from build123d import *

# Parameters (mm, degrees)
SKICA1_W                  = 100
SKICA1_H                  = 100
P_IDAT_VYSUNUT_M1_DEPTH   = 3
SKICA2_R                  = 1.5
ODEBRAT_VYSUNUT_M5_DEPTH  = 3
SKICA3_W                  = 75
SKICA3_H                  = 2
P_IDAT_VYSUNUT_M4_DEPTH   = 53
SKICA10_W                 = 8
SKICA10_H                 = 2
ODEBRAT_VYSUNUT_M6_DEPTH  = 50
SKICA11_W                 = 10
SKICA11_H                 = 2
ODEBRAT_VYSUNUT_M8_DEPTH  = 15
SKICA16_W                 = 67
SKICA16_H                 = 2
P_IDAT_VYSUNUT_M6_DEPTH   = 15
SKICA17_W                 = 2.5
SKICA17_H                 = 2.5
P_IDAT_VYSUNUT_M7_DEPTH   = 15
SKICA18_W                 = 2.5
SKICA18_H                 = 2.5
P_IDAT_VYSUNUT_M8_DEPTH   = 15
SKICA19_W                 = 1
SKICA19_H                 = 1
P_IDAT_VYSUNUT_M10_DEPTH  = 50
SKICA20_W                 = 1
SKICA20_H                 = 1
P_IDAT_VYSUNUT_M11_DEPTH  = 35
SKICA21_W                 = 1
SKICA21_H                 = 1
P_IDAT_VYSUNUT_M12_DEPTH  = 35
SKICA22_W                 = 1
SKICA22_H                 = 1
P_IDAT_VYSUNUT_M13_DEPTH  = 50
SKICA24_W                 = 91
SKICA24_H                 = 2
P_IDAT_VYSUNUT_M14_DEPTH  = 15
SKICA25_W                 = 2
SKICA25_H                 = 2
P_IDAT_VYSUNUT_M15_DEPTH  = 35
SKICA26_W                 = 2
SKICA26_H                 = 2
P_IDAT_VYSUNUT_M16_DEPTH  = 35
SKICA27_W                 = 2
SKICA27_H                 = 49.75
P_IDAT_VYSUNUT_M17_DEPTH  = 15
SKICA28_W                 = 100
SKICA28_H                 = 5
P_IDAT_VYSUNUT_M18_DEPTH  = 5
SKICA30_W                 = 5
SKICA30_H                 = 90
P_IDAT_VYSUNUT_M19_DEPTH  = 5
SKICA31_W                 = 100
SKICA31_H                 = 100
ODEBRAT_VYSUNUT_M9_DEPTH  = 6
SKICA32_W                 = 2
SKICA32_H                 = 15
ODEBRAT_VYSUNUT_M10_DEPTH = 6
SKICA33_W                 = 2
SKICA33_H                 = 23
P_IDAT_VYSUNUT_M22_DEPTH  = 25
P_IDAT_VYSUNUT_M23_DEPTH  = 10
SKICA35_W                 = 50
SKICA35_H                 = 2
P_IDAT_VYSUNUT_M24_DEPTH  = 10
SKICA36_W                 = 2
SKICA36_H                 = 45
P_IDAT_VYSUNUT_M25_DEPTH  = 2
SKICA37_W                 = 2
SKICA37_H                 = 2
P_IDAT_VYSUNUT_M26_DEPTH  = 60
SKICA38_W                 = 10
SKICA38_H                 = 1
P_IDAT_VYSUNUT_M27_DEPTH  = 35
SKICA40_W                 = 2
SKICA40_H                 = 2
P_IDAT_VYSUNUT_M29_DEPTH  = 35


with BuildPart() as part:
    # Skica1 → Přidat vysunutím1 (new body)
    with BuildSketch(Plane(origin=(0, 0, 0), x_dir=(1, 0, 0), z_dir=(0, 1, 0))):
        Rectangle(SKICA1_W, SKICA1_H)
    extrude(amount=P_IDAT_VYSUNUT_M1_DEPTH)

    # Skica2 → Odebrat vysunutím5 (cut)
    with BuildSketch(Plane(origin=(0, 0, 0), x_dir=(1, 0, 0), z_dir=(0, 1, 0))):
        with Locations((-18, 40)):
            Circle(SKICA2_R)
        with Locations((40, 40)):
            Circle(SKICA2_R)
        with Locations((40, -8.5)):
            Circle(SKICA2_R)
        with Locations((-18, -8.5)):
            Circle(SKICA2_R)
    extrude(amount=ODEBRAT_VYSUNUT_M5_DEPTH, mode=Mode.SUBTRACT)

    # Skica3 → Přidat vysunutím4 (add)
    with BuildSketch(Plane(origin=(0, 0, 0), x_dir=(1, 0, 0), z_dir=(0, 1, 0))):
        Polygon((40, 50), (40, 48), (48, 48), (48, 27.25), (50, 27.25), (50, 50), align=None)
        Polygon((-50, -20), (-48, -20), (-48, -48), (48, -48), (48, 4.25), (50, 4.25), (50, -50), (-50, -50), align=None)
        with Locations((-12.5, 49)):
            Rectangle(SKICA3_W, SKICA3_H)
    extrude(amount=P_IDAT_VYSUNUT_M4_DEPTH)

    # Skica10 → Odebrat vysunutím6 (cut)
    with BuildSketch(Plane(origin=(0, 53, 0), x_dir=(1, 0, 0), z_dir=(0, 1, 0))):
        with Locations((21, 49)):
            Rectangle(SKICA10_W, SKICA10_H)
    extrude(amount=-ODEBRAT_VYSUNUT_M6_DEPTH, mode=Mode.SUBTRACT)

    # Skica11 → Odebrat vysunutím8 (cut)
    with BuildSketch(Plane(origin=(0, 53, 0), x_dir=(1, 0, 0), z_dir=(0, 1, 0))):
        with Locations((-32, -49)):
            Rectangle(SKICA11_W, SKICA11_H)
        with Locations((-11, -49)):
            Rectangle(SKICA11_W, SKICA11_H)
        with Locations((10, -49)):
            Rectangle(SKICA11_W, SKICA11_H)
        with Locations((31, -49)):
            Rectangle(SKICA11_W, SKICA11_H)
    extrude(amount=-ODEBRAT_VYSUNUT_M8_DEPTH, mode=Mode.SUBTRACT)

    # Skica16 → Přidat vysunutím6 (add)
    with BuildSketch(Plane(origin=(0, 3, 0), x_dir=(1, 0, 0), z_dir=(0, 1, 0))):
        with Locations((-16.5, 47)):
            Rectangle(SKICA16_W, SKICA16_H)
    extrude(amount=P_IDAT_VYSUNUT_M6_DEPTH)

    # Skica17 → Přidat vysunutím7 (add)
    with BuildSketch(Plane(origin=(0, 3, 0), x_dir=(1, 0, 0), z_dir=(0, 1, 0))):
        with Locations((46.75, -46.75)):
            Rectangle(SKICA17_W, SKICA17_H)
    extrude(amount=P_IDAT_VYSUNUT_M7_DEPTH)

    # Skica18 → Přidat vysunutím8 (add)
    with BuildSketch(Plane(origin=(0, 3, 0), x_dir=(1, 0, 0), z_dir=(0, 1, 0))):
        with Locations((-46.75, -46.75)):
            Rectangle(SKICA18_W, SKICA18_H)
    extrude(amount=P_IDAT_VYSUNUT_M8_DEPTH)

    # Skica19 → Přidat vysunutím10 (add)
    with BuildSketch(Plane(origin=(0, 3, 0), x_dir=(1, 0, 0), z_dir=(0, 1, 0))):
        with Locations((47.5, 47.5)):
            Rectangle(SKICA19_W, SKICA19_H)
    extrude(amount=P_IDAT_VYSUNUT_M10_DEPTH)

    # Skica20 → Přidat vysunutím11 (add)
    with BuildSketch(Plane(origin=(0, 18, 0), x_dir=(1, 0, 0), z_dir=(0, 1, 0))):
        with Locations((47.5, -47.5)):
            Rectangle(SKICA20_W, SKICA20_H)
    extrude(amount=P_IDAT_VYSUNUT_M11_DEPTH)

    # Skica21 → Přidat vysunutím12 (add)
    with BuildSketch(Plane(origin=(0, 18, 0), x_dir=(1, 0, 0), z_dir=(0, 1, 0))):
        with Locations((-47.5, -47.5)):
            Rectangle(SKICA21_W, SKICA21_H)
    extrude(amount=P_IDAT_VYSUNUT_M12_DEPTH)

    # Skica22 → Přidat vysunutím13 (add)
    with BuildSketch(Plane(origin=(0, 3, 0), x_dir=(1, 0, 0), z_dir=(0, 1, 0))):
        with Locations((-47.5, -20.5)):
            Rectangle(SKICA22_W, SKICA22_H)
    extrude(amount=P_IDAT_VYSUNUT_M13_DEPTH)

    # Skica24 → Přidat vysunutím14 (add)
    with BuildSketch(Plane(origin=(0, 3, 0), x_dir=(1, 0, 0), z_dir=(0, 1, 0))):
        with Locations((0, -47)):
            Rectangle(SKICA24_W, SKICA24_H)
    extrude(amount=P_IDAT_VYSUNUT_M14_DEPTH)

    # Skica25 → Přidat vysunutím15 (add)
    with BuildSketch(Plane(origin=(0, 18, 0), x_dir=(1, 0, 0), z_dir=(0, 1, 0))):
        with Locations((20.5, -47)):
            Rectangle(SKICA25_W, SKICA25_H)
        with Locations((-0.5, -47)):
            Rectangle(SKICA25_W, SKICA25_H)
        with Locations((-21.5, -47)):
            Rectangle(SKICA25_W, SKICA25_H)
    extrude(amount=P_IDAT_VYSUNUT_M15_DEPTH)

    # Skica26 → Přidat vysunutím16 (add)
    with BuildSketch(Plane(origin=(0, 18, 0), x_dir=(1, 0, 0), z_dir=(0, 1, 0))):
        with Locations((-49, 47)):
            Rectangle(SKICA26_W, SKICA26_H)
        with Locations((16, 47)):
            Rectangle(SKICA26_W, SKICA26_H)
    extrude(amount=P_IDAT_VYSUNUT_M16_DEPTH)

    # Skica27 → Přidat vysunutím17 (add)
    with BuildSketch(Plane(origin=(0, 3, 0), x_dir=(1, 0, 0), z_dir=(0, 1, 0))):
        with Locations((47, -20.625)):
            Rectangle(SKICA27_W, SKICA27_H)
    extrude(amount=P_IDAT_VYSUNUT_M17_DEPTH)

    # Skica28 → Přidat vysunutím18 (add)
    with BuildSketch(Plane(origin=(0, 0, 0), x_dir=(1, 0, 0), z_dir=(0, 1, 0))):
        with Locations((0, -47.5)):
            Rectangle(SKICA28_W, SKICA28_H)
        with Locations((0, 47.5)):
            Rectangle(SKICA28_W, SKICA28_H)
    extrude(amount=-P_IDAT_VYSUNUT_M18_DEPTH)

    # Skica30 → Přidat vysunutím19 (add)
    with BuildSketch(Plane(origin=(0, 0, 0), x_dir=(-1, 0, 0), z_dir=(0, -1, 0))):
        with Locations((47.5, 0)):
            Rectangle(SKICA30_W, SKICA30_H)
        with Locations((-47.5, 0)):
            Rectangle(SKICA30_W, SKICA30_H)
    extrude(amount=P_IDAT_VYSUNUT_M19_DEPTH)

    # Skica31 → Odebrat vysunutím9 (cut)
    with BuildSketch(Plane(origin=(0, -5, 0), x_dir=(-1, 0, 0), z_dir=(0, -1, 0))):
        Rectangle(SKICA31_W, SKICA31_H)
    extrude(amount=-ODEBRAT_VYSUNUT_M9_DEPTH, mode=Mode.SUBTRACT)

    # Skica32 → Odebrat vysunutím10 (cut)
    with BuildSketch(Plane.ZY.offset(-15)):
        with Locations((-47, 45.5)):
            Rectangle(SKICA32_W, SKICA32_H)
    extrude(amount=-ODEBRAT_VYSUNUT_M10_DEPTH, mode=Mode.SUBTRACT)

    # Skica33 → Přidat vysunutím22 (add)
    with BuildSketch(Plane(origin=(0, 3, 0), x_dir=(1, 0, 0), z_dir=(0, 1, 0))):
        with Locations((49, 15.75)):
            Rectangle(SKICA33_W, SKICA33_H)
    extrude(amount=P_IDAT_VYSUNUT_M22_DEPTH)

    # Skica34 → Přidat vysunutím23 (add)
    with BuildSketch(Plane(origin=(0, 53, 0), x_dir=(1, 0, 0), z_dir=(0, 1, 0))):
        Polygon((40, 50), (50, 50), (50, 27.25), (48, 27.25), (48, 47), (47, 47), (47, 48), (40, 48), align=None)
    extrude(amount=P_IDAT_VYSUNUT_M23_DEPTH)

    # Skica35 → Přidat vysunutím24 (add)
    with BuildSketch(Plane(origin=(0, 53, 0), x_dir=(1, 0, 0), z_dir=(0, 1, 0))):
        with Locations((-8, 49)):
            Rectangle(SKICA35_W, SKICA35_H)
    extrude(amount=P_IDAT_VYSUNUT_M24_DEPTH)

    # Skica36 → Přidat vysunutím25 (add)
    with BuildSketch(Plane.XY.offset(-48)):
        with Locations((-32, 40.5)):
            Rectangle(SKICA36_W, SKICA36_H)
    extrude(amount=P_IDAT_VYSUNUT_M25_DEPTH)

    # Skica37 → Přidat vysunutím26 (add)
    with BuildSketch(Plane(origin=(0, 3, 0), x_dir=(1, 0, 0), z_dir=(0, 1, 0))):
        with Locations((47, 38)):
            Rectangle(SKICA37_W, SKICA37_H)
    extrude(amount=P_IDAT_VYSUNUT_M26_DEPTH)

    # Skica38 → Přidat vysunutím27 (add)
    with BuildSketch(Plane(origin=(0, 3, 0), x_dir=(1, 0, 0), z_dir=(0, 1, 0))):
        with Locations((22, 49.5)):
            Rectangle(SKICA38_W, SKICA38_H)
    extrude(amount=P_IDAT_VYSUNUT_M27_DEPTH)

    # Skica40 → Přidat vysunutím29 (add)
    with BuildSketch(Plane(origin=(0, 53, 0), x_dir=(1, 0, 0), z_dir=(0, 1, 0))):
        with Locations((47, -6.75)):
            Rectangle(SKICA40_W, SKICA40_H)
    extrude(amount=-P_IDAT_VYSUNUT_M29_DEPTH)


solid = part.part
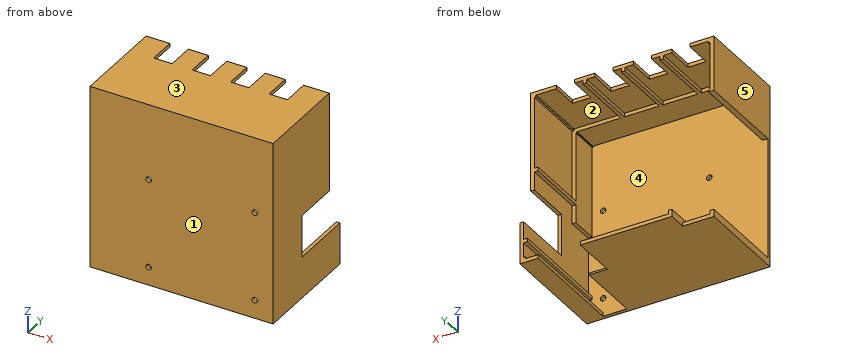
Can you work these out from the model? Positions are in its coordinate system, mm. Face numbers are marked on the shaded views. A direction names the side the tool comes from. Coordinates: 2 decimals unless noted, no trailing zeros. Write each loop counter-clockwise with the first axis right and the second up, starting at its lowest first coordinate (ties: lowest second). Pieces come first, ordered by that corner, then holes. Notation, with made-up numbers: (-17.75, 8) -> (20.25, 8) arc R18 ccw to (20.25, 28) -> close; hole circle Ø11 at (63, -21.5). An arc over 180 degrees is marked (long way). Write item = value, one per line.
(1) On a 3-axis mill with a long thin cutter (end or side, diameter ignored), from which of +Z, -Z, +X, -X, +Y, -Y can I reach the whole of each face in a straight line? I mean the marked faces 1 and 2. Say none if no direction works.
Verdict:
face_1 = +Z, -Z, +X, -X, -Y
face_2 = +Y
(2) Imagine slicing it at D-D (x = 9). Please give me the cut outline in (y, z), and give its area (3 significant figures).
Verdict:
outline = (1, -50) -> (63, -50) -> (63, -48) -> (18, -48) -> (18, -46) -> (3, -46) -> (3, 46) -> (18, 46) -> (18, 48) -> (38, 48) -> (38, 50) -> (1, 50) -> close
area = 450 mm^2
(3) Imagine slicing it at C-C (z = 40.5). Please give me the cut outline in (x, y), and give its area (3 significant figures).
Verdict:
outline = (-50, 1) -> (50, 1) -> (50, 53) -> (48, 53) -> (48, 18) -> (46, 18) -> (46, 3) -> (-48, 3) -> (-48, 53) -> (-50, 53) -> close
area = 430 mm^2
(4) For pin 1 (8 mm diameter, centred on y = 35.5, z = -18, fed in from -X); pin 2 (14.5 mm diameter, centred on x = -44, z = 34.5, fed in from +Y); pin 3 (2 mm diameter, centred on x = 32.5, z = 49, fed in from +Y); pin 4 (1 mm diameter, centred on x = -5.5, z = -47, fed in from +Y), each with a flat end and sliding along its axis, tell me the tip position at first contact or that it passes through.
Verdict:
pin_1 = through
pin_2 = 53
pin_3 = 38
pin_4 = 18
(5) Imagine slicing it at A-A (x = -18). Please give me the cut outline in (y, z).
Verdict:
outline = (1, -50) -> (63, -50) -> (63, -48) -> (18, -48) -> (18, -46) -> (3, -46) -> (3, -41.5) -> (1, -41.5) -> close; (1, -38.5) -> (3, -38.5) -> (3, 7) -> (1, 7) -> close; (1, 10) -> (3, 10) -> (3, 46) -> (18, 46) -> (18, 48) -> (53, 48) -> (53, 50) -> (1, 50) -> close
(6) If I drill on probe 1 along X at (y, z) = (2.4, 8.5); probe 2 along Z at (x, y) = (40, 2); probe 3 along Z at (x, y) = (1.5, 23), over which ranges is the centre line in solid material (lowest first)?
Verdict:
probe_1 = -50 to -19.5, -16.5 to 38.5, 41.5 to 50
probe_2 = -50 to -41.5, -38.5 to 7, 10 to 50
probe_3 = -50 to -48, 48 to 50
(7) Thinking about a two-plate mould opening in Z: for the marked faces 3, 4 and 5, which applies, +Z half, -Z half, draft (parallel to the pull), parting line (faces both ways), or undercut?
Verdict:
face_3 = +Z half
face_4 = undercut
face_5 = draft
